Design review of the part shown in the three views and the two pictorial views. Dimensions are in mm from the part's minimum x, y and z. A direction names the side the tool comes from. Coordinates: 2 decimals unless noted, no trailing zeros. Loops run counter-clockwise (first coordinate to the right, second up) from the corner with the lowest first, then second, coordinate; pieces in that order, holes last. Notation, with made-up numbers: M 15,-1.5 L 37,-1.5 A19 cw 37,8.5 Z; hole C 14.25,16 d4. An arc over 180 degrees is marked long. Use one line per item in the form item = value.
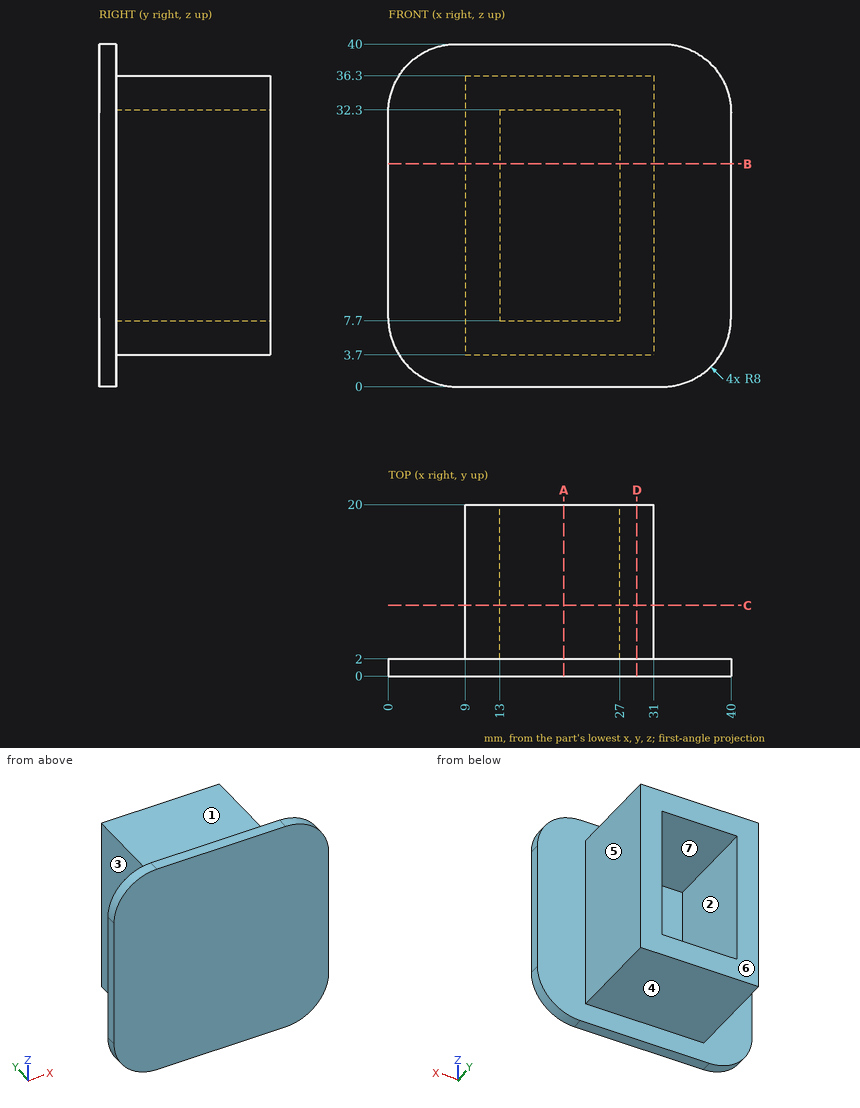
1. Add section A-A (x = 20.5). State the section outline as (y, z) points.
Response values:
outline = M 0,0 L 2,0 L 2,3.7 L 20,3.7 L 20,7.7 L 2,7.7 L 2,32.3 L 20,32.3 L 20,36.3 L 2,36.3 L 2,40 L 0,40 Z
2. Add section D-D (x = 29). State the section outline as (y, z) points.
Response values:
outline = M 0,0 L 2,0 L 2,3.7 L 20,3.7 L 20,36.3 L 2,36.3 L 2,40 L 0,40 Z
3. Wall thickness on line 1 along X through (y, z) = (17.5, 8.5); line 2 along Z through (x, y) = (17, 14.75); line 3 along Y through (x, z) = (32.5, 21): over which ranges is each line inside the solid? List them lowest first. Write a range as from..to.
Response values:
line_1 = 9..13, 27..31
line_2 = 3.7..7.7, 32.3..36.3
line_3 = 0..2
4. Add section B-B (z = 26). State the section outline as (x, y) points, then the cut area to 3 significant figures.
Response values:
outline = M 0,0 L 40,0 L 40,2 L 31,2 L 31,20 L 27,20 L 27,2 L 13,2 L 13,20 L 9,20 L 9,2 L 0,2 Z
area = 224 mm^2
5. Insertion check: P1, Ø2, axis at x = 25, y = 6.5, coming from the +Z side; P2, Ø5.5, axis at y = 15, z = 15, coming from the -X side; P3, Ø9, axis at x = 23, y = 14, coming from the -Z side. Each pin has a flat end and moves straight along its axis. Give the tip position at first contact, or say it passes through.
Response values:
P1 = 36.3
P2 = 9
P3 = 3.7
6. Add section C-C (y = 8.25). State the section outline as (x, z) points.
Response values:
outline = M 9,3.7 L 31,3.7 L 31,36.3 L 9,36.3 Z; hole M 13,7.7 L 27,7.7 L 27,32.3 L 13,32.3 Z
7. Machinability: for the marked faces 1, 2, 3 and 4, which of the approach directions +Z, -Z, +X, -X, +Y, -Y give a long, thin tool a straight path to every point of the face, cutting with its end or side? Answer none if there is none.
Response values:
face_1 = +Z, +X, -X, +Y
face_2 = +Y
face_3 = +Z, -Z, -X, +Y
face_4 = -Z, +X, -X, +Y
8. The part is to be moulded in two halves that separate along X. For the marked faces 5, 6 and 7, say which applies: pulls with the +X half, pulls with the -X half, needs draft (parallel to the pull), parting line crosses it, or undercut.
Response values:
face_5 = pulls with the +X half
face_6 = needs draft
face_7 = undercut
